The listing builds one solid part. Answer for the finished solid, in the listing's coordinates (mm). A direction names the side the tool comes from. Coordinates: 2 decimals unless noted, no trailing zeros. Write each loop counter-clockwise with the first axis right and the second up, starting at its lowest first coordinate (ties: lowest second). Pieces come first, ordered by that corner, then holes.
(1) The part is cut by section B-B on z = -8.97. Determine the outline of the cut face in (x, y).
(2) The part is cut by section C-C on z = -38.87. Determine the outline of the cut face in (x, y).
(3) For a pull along Z with two mould halves and no side action, classify faces 5 (the flat face through (-26.495, 21, -39)), 6 (the flat face through (-76, 22, 0)), 7 (the flat face through (-54, 38, 0)) as +Z half, -Z half, draft (parallel to the pull), parting line (faces both ways), or undercut.
(4) The part is cut by section A-A on x = -50. Determine the outline of the cut face in (y, z), plus the area to 3 significant figures.
(5) The part is cut by section D-D on z = 24.5. Determine the outline of the cut face in (x, y).
(6) Given P1, Ø10, axis at y = 11, z = -35.5, coming from the -X side; P2, Ø3, axis at y = 8, z = -8.5, coming from the +X side; P3, Ø1, axis at y = 37.5, z = 43.5, coming from the -X side, each flat-ended and moving along its own axis, determine where each tip first touches the part or whether it passes through.
(7) Straight lines are drawn through the part: line 1 (Y direction, x = -68.55, z = -48.85); line 2 (Y direction, x = -50.5, z = -48.78); line 3 (X direction, y = 6, z = -33.5). For each, find the intervals that lie inside material, in ascending order.
(8) Which of the six approach directions +Z, -Z, +X, -X, +Y, -Y give full straight-line access (tool end or side, diameter ignored) to faces 1 (the cylindrical face through (-69.83, 8.25, -8.21)), 2 (the flat face through (-59, 41.836, -29)), 3 (the flat face through (-76.295, 21, -38)), 4 (the flat face through (-55.495, 8, -49))?
from build123d import *

# Parameters (mm, degrees)
SKETCH4_R           = 18.6
BOSS_EXTRUDE3_DEPTH = 76.2
SKETCH5_R           = 0.75
BOSS_EXTRUDE4_DEPTH = 15
SKETCH6_R           = 0.75
BOSS_EXTRUDE5_DEPTH = 15
SKETCH7_W           = 26.8
SKETCH7_H           = 40
BOSS_EXTRUDE6_DEPTH = 58
SKETCH8_R           = 1.75
CUT_EXTRUDE1_DEPTH  = 5
SKETCH9_R           = 1.75
CUT_EXTRUDE2_DEPTH  = 5
SKETCH10_R          = 1.75
CUT_EXTRUDE3_DEPTH  = 5
SKETCH11_R          = 1.75
CUT_EXTRUDE4_DEPTH  = 5
SKETCH12_R          = 9.4
BOSS_EXTRUDE7_DEPTH = 4
SKETCH13_R          = 1.75
CUT_EXTRUDE5_DEPTH  = 10
SKETCH14_R          = 1.75
CUT_EXTRUDE6_DEPTH  = 10
SKETCH17_R          = 1.75
CUT_EXTRUDE7_DEPTH  = 10
SKETCH18_R          = 1.75
CUT_EXTRUDE8_DEPTH  = 10
SKETCH19_R          = 9.315
BOSS_EXTRUDE8_DEPTH = 4
SKETCH21_R          = 3.5
BOSS_EXTRUDE9_DEPTH = 15


with BuildPart() as part:
    # Sketch4 → Boss-Extrude3 (new body)
    with BuildSketch(Plane.XY):
        with Locations(Location((-63.856856352, 21.865677116, 0), (0, 0, 180))):
            Circle(SKETCH4_R)
    extrude(amount=BOSS_EXTRUDE3_DEPTH)

    # Sketch5 → Boss-Extrude4 (add)
    with BuildSketch(Plane.XY.offset(76.2)):
        with Locations((-66.305296551, 38.820097555)):
            Circle(SKETCH5_R)
    extrude(amount=BOSS_EXTRUDE4_DEPTH)

    # Sketch6 → Boss-Extrude5 (add)
    with BuildSketch(Plane.XY.offset(76.2)):
        with Locations((-69.224873833, 38.364991381)):
            Circle(SKETCH6_R)
    extrude(amount=BOSS_EXTRUDE5_DEPTH)

    # Sketch7 → Boss-Extrude6 (add)
    with BuildSketch(Plane(origin=(0, 0, 0), x_dir=(-1, 0, 0), z_dir=(0, 0, -1))):
        with Locations((58.895304338, 21.83595021)):
            Rectangle(SKETCH7_W, SKETCH7_H)
    extrude(amount=BOSS_EXTRUDE6_DEPTH)

    # Sketch8 → Cut-Extrude1 (cut)
    with BuildSketch(Plane.ZY.offset(72.295304338)):
        with Locations((-48.85, 35.53595021)):
            Circle(SKETCH8_R)
    extrude(amount=-CUT_EXTRUDE1_DEPTH, mode=Mode.SUBTRACT)

    # Sketch9 → Cut-Extrude2 (cut)
    with BuildSketch(Plane.ZY.offset(72.295304338)):
        with Locations((-9.15, 35.53595021)):
            Circle(SKETCH9_R)
    extrude(amount=-CUT_EXTRUDE2_DEPTH, mode=Mode.SUBTRACT)

    # Sketch10 → Cut-Extrude3 (cut)
    with BuildSketch(Plane.ZY.offset(72.295304338)):
        with Locations((-48.85, 6.77595021)):
            Circle(SKETCH10_R)
    extrude(amount=-CUT_EXTRUDE3_DEPTH, mode=Mode.SUBTRACT)

    # Sketch11 → Cut-Extrude4 (cut)
    with BuildSketch(Plane.ZY.offset(72.295304338)):
        with Locations((-9.15, 6.77595021)):
            Circle(SKETCH11_R)
    extrude(amount=-CUT_EXTRUDE4_DEPTH, mode=Mode.SUBTRACT)

    # Sketch12 → Boss-Extrude7 (add)
    with BuildSketch(Plane.ZY.offset(72.295304338)):
        with Locations(Location((-38.6, 21.23595021, 0), (0, 0, 180))):
            Circle(SKETCH12_R)
    extrude(amount=BOSS_EXTRUDE7_DEPTH)

    # Sketch13 → Cut-Extrude5 (cut)
    with BuildSketch(Plane(origin=(-45.495304338, 0, 0), x_dir=(0, 0, -1), z_dir=(1, 0, 0))):
        with Locations((8.97, 35.91595021)):
            Circle(SKETCH13_R)
    extrude(amount=-CUT_EXTRUDE5_DEPTH, mode=Mode.SUBTRACT)

    # Sketch14 → Cut-Extrude6 (cut)
    with BuildSketch(Plane(origin=(-45.495304338, 0, 0), x_dir=(0, 0, -1), z_dir=(1, 0, 0))):
        with Locations((8.97, 8.06595021)):
            Circle(SKETCH14_R)
    extrude(amount=-CUT_EXTRUDE6_DEPTH, mode=Mode.SUBTRACT)

    # Sketch17 → Cut-Extrude7 (cut)
    with BuildSketch(Plane(origin=(-45.495304338, 0, 0), x_dir=(0, 0, -1), z_dir=(1, 0, 0))):
        with Locations((48.78, 8.26595021)):
            Circle(SKETCH17_R)
    extrude(amount=-CUT_EXTRUDE7_DEPTH, mode=Mode.SUBTRACT)

    # Sketch18 → Cut-Extrude8 (cut)
    with BuildSketch(Plane(origin=(-45.495304338, 0, 0), x_dir=(0, 0, -1), z_dir=(1, 0, 0))):
        with Locations((48.88, 35.40595021)):
            Circle(SKETCH18_R)
    extrude(amount=-CUT_EXTRUDE8_DEPTH, mode=Mode.SUBTRACT)

    # Sketch19 → Boss-Extrude8 (add)
    with BuildSketch(Plane(origin=(-45.495304338, 0, 0), x_dir=(0, 0, -1), z_dir=(1, 0, 0))):
        with Locations(Location((38.87, 20.96595021, 0), (0, 0, 180))):
            Circle(SKETCH19_R)
    extrude(amount=BOSS_EXTRUDE8_DEPTH)

    # Sketch21 → Boss-Extrude9 (add)
    with BuildSketch(Plane(origin=(-41.495304338, 0, 0), x_dir=(0, 0, -1), z_dir=(1, 0, 0))):
        with Locations((38.87, 20.96595021)):
            Circle(SKETCH21_R)
    extrude(amount=BOSS_EXTRUDE9_DEPTH)


solid = part.part
Model answer:
1. outline: (-72.3, 1.84) - (-45.5, 1.84) - (-45.5, 6.32) - (-55.5, 6.32) - (-55.5, 9.82) - (-45.5, 9.82) - (-45.5, 34.17) - (-55.5, 34.17) - (-55.5, 37.67) - (-45.5, 37.67) - (-45.5, 41.84) - (-72.3, 41.84) - (-72.3, 37.28) - (-67.3, 37.28) - (-67.3, 33.8) - (-72.3, 33.8) - (-72.3, 8.52) - (-67.3, 8.52) - (-67.3, 5.04) - (-72.3, 5.04) - close
2. outline: (-76.3, 11.84) - (-72.3, 11.84) - (-72.3, 1.84) - (-45.5, 1.84) - (-45.5, 11.65) - (-41.5, 11.65) - (-41.5, 17.47) - (-26.5, 17.47) - (-26.5, 24.47) - (-41.5, 24.47) - (-41.5, 30.28) - (-45.5, 30.28) - (-45.5, 41.84) - (-72.3, 41.84) - (-72.3, 30.63) - (-76.3, 30.63) - close
3. face 5: draft
3. face 6: undercut
3. face 7: +Z half
4. outline: (1.84, -58) - (41.84, -58) - (41.84, 0) - (34.27, 0) - (34.27, 76.2) - (9.46, 76.2) - (9.46, 0) - (1.84, 0) - close; hole circle Ø3.5 at (8.07, -8.97); hole circle Ø3.5 at (8.27, -48.78); hole circle Ø3.5 at (35.41, -48.88); hole circle Ø3.5 at (35.92, -8.97)
4. area: 4,170 mm2
5. outline: circle Ø37.2 at (-63.86, 21.87)
6. P1: stops at x = -76.3
6. P2: stops at x = -45.5
6. P3: stops at x = -74.67
7. line 1: y = 1.84 to 5.03, 8.53 to 33.79, 37.29 to 41.84
7. line 2: y = 1.84 to 6.52, 10.02 to 33.66, 37.15 to 41.84
7. line 3: x = -72.3 to -45.5
8. face 1: -X
8. face 2: +Z, -Z, +X, -X, +Y
8. face 3: -Z, -X, +Y, -Y
8. face 4: +X
